```python
from build123d import *

# Parameters (mm, degrees)
CUT_EXTRUDE2_DEPTH = 1.54


with BuildPart() as part:
    # Sketch10 → Revolve3 (revolve)
    with BuildSketch(Plane(origin=(0, 0, 0), x_dir=(0, 0, -1), z_dir=(1, 0, 0)), mode=Mode.PRIVATE) as revolve3_sk:
        Polygon((13.675, 2), (14.2, 1.475), (14.2, 0), (2.2, 0), (2.2, 2), align=None)
    revolve(revolve3_sk.sketch.rotate(Axis((0, 0, 0), (0, 0, -1)), 90), axis=Axis((0, 0, 0), (0, 0, -1)))

    # Sketch7 → Revolve2 (revolve)
    with BuildSketch(Plane(origin=(0, 0, 0), x_dir=(0, 0, -1), z_dir=(1, 0, 0)), mode=Mode.PRIVATE) as revolve2_sk:
        with BuildLine():
            Line((1.87, 3.8), (2.2, 3.8))
            Line((2.2, 3.8), (2.2, 0))
            Line((2.2, 0), (0, 0))
            Line((0, 0), (0, 2))
            ThreePointArc((0, 2), (0.793500147, 3.047002626), (1.87, 3.8))
        make_face()
    revolve(revolve2_sk.sketch.rotate(Axis((0, 0, 0), (0, 0, -1)), 180), axis=Axis((0, 0, 0), (0, 0, -1)))

    # Sketch5 → Cut-Extrude2 (cut)
    with BuildSketch(Plane.XY):
        Polygon((1.25, -0.721687836), (1.25, 0.721687836), (0, 1.443375673), (-1.25, 0.721687836), (-1.25, -0.721687836), (0, -1.443375673), align=None)
    extrude(amount=-CUT_EXTRUDE2_DEPTH, mode=Mode.SUBTRACT)

    # Cut-Extrude3 cone 1 section (through the dimple's axis) → Cut-Extrude3 (revolve, cut)
    with BuildSketch(Plane(origin=(0, 0, 0), x_dir=(0, -1, 0), z_dir=(1, 0, 0))):
        Polygon((0, 0), (1.443375673, 0), (0, 1.443375673), align=None)
    revolve(axis=Axis((0, 0, 0), (0, 0, -1)), mode=Mode.SUBTRACT)


with BuildPart() as body_2:
    # Split1: read off the stored shape, not the designer's step
    # Split1: the piece on the far side of the plane
    add(part.part)
    split(bisect_by=Plane.XY.offset(-2.2), keep=Keep.BOTTOM)


with BuildPart() as part_1:
    add(part.part)

    # Split1
    split(bisect_by=Plane.XY.offset(-2.2), keep=Keep.TOP)


with BuildPart() as body_2_1:
    add(body_2.part)

    # Boss-Extrude1: read off the stored shape, not the designer's step
    # Boss-Extrude1: union part
    add(part_1.part)


solid = body_2_1.part
```
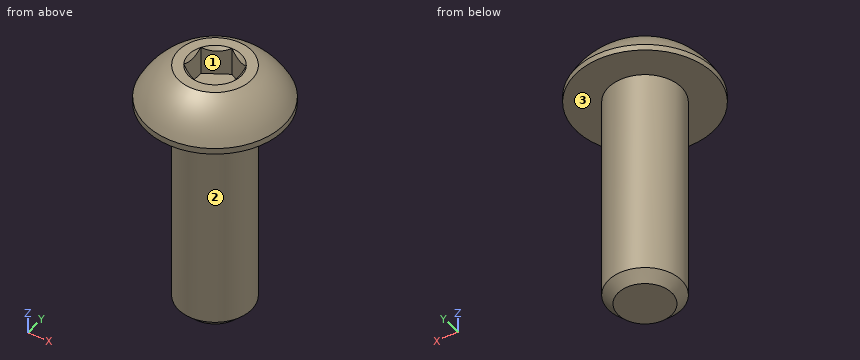
Verification items for the finished model (mm, model axes). Face numbers are marked on the shaded views. Round coordinates to 2 decimals unless told otherwise and drop trailing zeros. Write each loop counter-clockwise with the first axis right and the second up, starting at its lowest first coordinate (ties: lowest second). Pieces come first, ordered by that corner, then holes.
1. Section check D-D on y = -2.5. Enter the section's corners in (x, z), plus the area to 3 significant figures.
2. Section check A-A on y = 0. Enter the section's corners in (x, z) (3 decimals), plus the area to 3 significant figures.
3. Section check B-B on z = -12.75. Enter the section's corners in (x, y), plus the area to 3 significant figures.
4. Section check C-C on x = 3. Enter the section's corners in (y, z), plus the area to 3 significant figures.
5. Scan lines: L1, parallel to Z at x = 2.25, y = 2.5; L2, parallel to X at y = 0.25, z = -5; L3, parallel to Z at x = -0.75, y = 1.75. Record each from-to range of solid material in increasing order.
6. Gauge pin test, flat ends, axial feed: P1, Ø3, axis at x = -3, y = 0, coming from the -Z side (3 decimals); P2, Ø1.5, axis at x = 1.5, y = -2, coming from the +Z side; P3, Ø2, axis at x = -0.5, z = -11, coming from the -Y side; P4, Ø3, axis at x = -2.5, z = -7, coming from the -Y side. Record the tip position at first contact, or that the pin passes through.
7. Draft check along X on the marked faces 1, 2 and 3. Enter one of: +X half, -X half, draft (parallel to the pull), parting line (faces both ways), or undercut.
Answer:
1. outline: (-2.86, -2.2) - (2.86, -2.2) - (2.86, -1.87) arc R3.41 ccw to (-2.86, -1.87) - close
1. area: 8.16 mm2
2. outline: (-3.8, -2.2) - (-2, -2.2) - (-2, -13.675) - (-1.475, -14.2) - (1.475, -14.2) - (2, -13.675) - (2, -2.2) - (3.8, -2.2) - (3.8, -1.87) arc R4.229 ccw to (2, 0) - (1.443, 0) - (1.25, -0.193) - (1.25, -1.54) - (-1.25, -1.54) - (-1.25, -0.193) - (-1.443, 0) - (-2, 0) arc R4.229 ccw to (-3.8, -1.87) - close
2. area: 57.9 mm2
3. outline: circle Ø4 at (0, 0)
3. area: 12.6 mm2
4. outline: (-2.33, -2.2) - (2.33, -2.2) - (2.33, -1.87) arc R2.98 ccw to (-2.33, -1.87) - close
4. area: 5.19 mm2
5. L1: z = -2.2 to -1.16
5. L2: x = -1.98 to 1.98
5. L3: z = -13.77 to 0
6. P1: stops at z = -14.175
6. P2: stops at z = 0
6. P3: stops at y = -2
6. P4: stops at y = -1.73
7. face 1: undercut
7. face 2: parting line
7. face 3: draft
